Check sheet for the modelled part. Datum: model origin and axes. Units: mm. Face numbers are marked on the shaded views. Coordinates: 2 decimals unless noted, no trailing zeros. Loops run counter-clockwise (first coordinate to the right, second up) from the corner with the lowest first, then second, coordinate; pieces in that order, holes last. Notation, with made-up numbers: M -1.75,-32 L 31.25,-32 A7 cw 31.25,-20 Z; hole C -6,0.25 d1. An arc over 180 degrees is marked long. Write each question's results on one line, items separated by ' | '. Start each with the question number.
from build123d import *

# Parameters (mm, degrees)
EXTRUDE_START             = -30
SKETCH_1_W                = 70
SKETCH_1_H                = 6
EXTRUDE_250_DEPTH         = 60
EXTRUDE_START_2           = -16.3
SKETCH_2_W                = 30
SKETCH_2_H                = 60
EXTRUDE_16_3_DEPTH        = 6
EXTRUDE_START_3           = 10.3
SKETCH_3_W                = 30
SKETCH_3_H                = 60
EXTRUDE_10_3_DEPTH        = 6
CUT_EXTRUDE_M4_DEPTH      = 103.95630141
CUT_EXTRUDE_M4_DEPTH_BACK = 103.95630141
SKETCH_4_R                = 2.25
F_6MM_START               = -46
SKETCH_5_R                = 2.7
F_6MM_DEPTH               = 6
F_21X13P5_DEPTH           = 106.432442825
F_21X13P5_DEPTH_BACK      = 106.432442825
SKETCH_6_R                = 1.4


with BuildPart() as part:
    # 草图1 → Extrude 250 (new body)
    with BuildSketch(Plane.XY.offset(EXTRUDE_START)):
        with Locations((55, -37)):
            Rectangle(SKETCH_1_W, SKETCH_1_H)
    extrude(amount=EXTRUDE_250_DEPTH)

    # 草图2 → 夹臂侧板-16.3 (add)
    with BuildSketch(Plane.XY.offset(EXTRUDE_START_2)):
        with Locations((15, -10)):
            Rectangle(SKETCH_2_W, SKETCH_2_H)
    extrude(amount=EXTRUDE_16_3_DEPTH)

    # 草图3 → 夹臂侧板10.3 (add)
    with BuildSketch(Plane.XY.offset(EXTRUDE_START_3)):
        with Locations((15, -10)):
            Rectangle(SKETCH_3_W, SKETCH_3_H)
    extrude(amount=EXTRUDE_10_3_DEPTH)

    # 草图4 → 夹臂M4通孔 (cut, two sides: drawn at the far end of the back side and taken through both)
    with BuildSketch(Plane.XY.offset(-CUT_EXTRUDE_M4_DEPTH_BACK)):
        with Locations(Location((12, -10, 0), (0, 0, 180))):
            Circle(SKETCH_4_R)
        with Locations(Location((12, 10, 0), (0, 0, 180))):
            Circle(SKETCH_4_R)
    extrude(amount=CUT_EXTRUDE_M4_DEPTH + CUT_EXTRUDE_M4_DEPTH_BACK, mode=Mode.SUBTRACT)

    # 草图5 → 相机6mm绝缘支柱 (add)
    with BuildSketch(Plane(origin=(0, 0, 0), x_dir=(1, 0, 0), z_dir=(0, 1, 0)).offset(F_6MM_START)):
        with Locations(Location((53.25, -10.5, 0), (0, 0, 270))):
            Circle(SKETCH_5_R)
        with Locations(Location((53.25, 10.5, 0), (0, 0, 270))):
            Circle(SKETCH_5_R)
        with Locations(Location((66.75, -10.5, 0), (0, 0, 270))):
            Circle(SKETCH_5_R)
        with Locations(Location((66.75, 10.5, 0), (0, 0, 270))):
            Circle(SKETCH_5_R)
    extrude(amount=F_6MM_DEPTH)

    # 草图6 → 21x13p5相机孔阵 (cut, two sides: drawn at the far end of the back side and taken through both)
    with BuildSketch(Plane(origin=(0, 0, 0), x_dir=(1, 0, 0), z_dir=(0, 1, 0)).offset(-F_21X13P5_DEPTH_BACK)):
        with Locations(Location((53.25, -10.5, 0), (0, 0, 270))):
            Circle(SKETCH_6_R)
        with Locations(Location((53.25, 10.5, 0), (0, 0, 270))):
            Circle(SKETCH_6_R)
        with Locations(Location((66.75, -10.5, 0), (0, 0, 270))):
            Circle(SKETCH_6_R)
        with Locations(Location((66.75, 10.5, 0), (0, 0, 270))):
            Circle(SKETCH_6_R)
    extrude(amount=F_21X13P5_DEPTH + F_21X13P5_DEPTH_BACK, mode=Mode.SUBTRACT)


solid = part.part
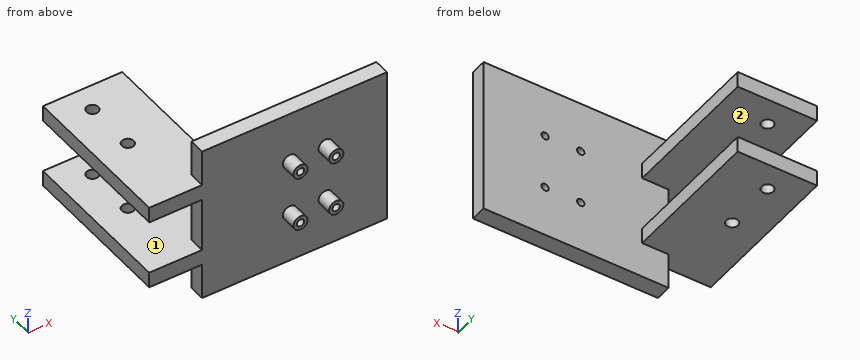
1) Gauge pin test, flat ends, axial feed: P1, Ø2, axis at x = 50, z = 8.5, coming from the +Y side; P2, Ø4, axis at y = -9, z = -12, coming from the +X side; P3, Ø3, axis at x = 19, y = -13.5, coming from the +Z side; P4, Ø4, axis at x = 12, y = -10, coming from the -Z side. Record the tip position at first contact, or that the pin passes through.
2) Section check A-A (y = -10). Enter the section's corners in (x, z).
3) Section check D-D (y = -17). Enter the section's corners in (x, z), then the cut area to 3 significant figures.
4) Section check C-C (x = 66.75). Enter the section's corners in (y, z).
5) Thickness scan on probe 1 along Z at (x, y) = (66.75, -39.25); probe 2 along X at (y, z) = (-40.5, -10.5); probe 3 along Y at (x, z) = (12, 11.9). Record the ranges inside material, lowest first.
6) Release check for a two-part mould opening along Z. For the marked faces 1 and 2 record: +Z half, -Z half, draft (parallel to the pull), parting line (faces both ways), or undercut.
7) Section check B-B (x = 12). Enter the section's corners in (y, z).
Return value:
1) P1: stops at y = -34 | P2: stops at x = 30 | P3: stops at z = 16.3 | P4: passes through
2) outline: M 0,-16.3 L 9.75,-16.3 L 9.75,-10.3 L 0,-10.3 Z; M 0,10.3 L 9.75,10.3 L 9.75,16.3 L 0,16.3 Z; M 14.25,-16.3 L 30,-16.3 L 30,-10.3 L 14.25,-10.3 Z; M 14.25,10.3 L 30,10.3 L 30,16.3 L 14.25,16.3 Z
3) outline: M 0,-16.3 L 30,-16.3 L 30,-10.3 L 0,-10.3 Z; M 0,10.3 L 30,10.3 L 30,16.3 L 0,16.3 Z | area: 360 mm2
4) outline: M -46,-13.2 L -40,-13.2 L -40,-30 L -34,-30 L -34,-11.9 L -46,-11.9 Z; M -46,-9.1 L -34,-9.1 L -34,9.1 L -46,9.1 L -46,7.8 L -40,7.8 L -40,-7.8 L -46,-7.8 Z; M -46,11.9 L -34,11.9 L -34,30 L -40,30 L -40,13.2 L -46,13.2 Z
5) probe 1: z = -30 to -11.9, -9.1 to 9.1, 11.9 to 30 | probe 2: x = 50.55 to 51.85, 54.65 to 55.95, 64.05 to 65.35, 68.15 to 69.45 | probe 3: y = -40 to -12.25, -7.75 to 7.75, 12.25 to 20
6) face 1: undercut | face 2: undercut
7) outline: M -40,-16.3 L -12.25,-16.3 L -12.25,-10.3 L -40,-10.3 Z; M -40,10.3 L -12.25,10.3 L -12.25,16.3 L -40,16.3 Z; M -7.75,-16.3 L 7.75,-16.3 L 7.75,-10.3 L -7.75,-10.3 Z; M -7.75,10.3 L 7.75,10.3 L 7.75,16.3 L -7.75,16.3 Z; M 12.25,-16.3 L 20,-16.3 L 20,-10.3 L 12.25,-10.3 Z; M 12.25,10.3 L 20,10.3 L 20,16.3 L 12.25,16.3 Z
